Source: three-view drawing plus pictorial views. Frame: mm from the lowest corner of the part. A direction names the side the tool comes from. Give positions to 0.01 mm unless a question says otherwise; leave off trailing zeros. Loops run counter-clockwise (first coordinate to the right, second up) from the corner with the lowest first, then second, coordinate; pieces in that order, holes last. Notation, with made-up numbers: (65.25, -34) - (113.25, -34) arc R19 cw to (113.25, 1) - close; hole circle Ø9 at (47, -31.75). An arc over 180 degrees is marked (long way). One line per item, written item: value.
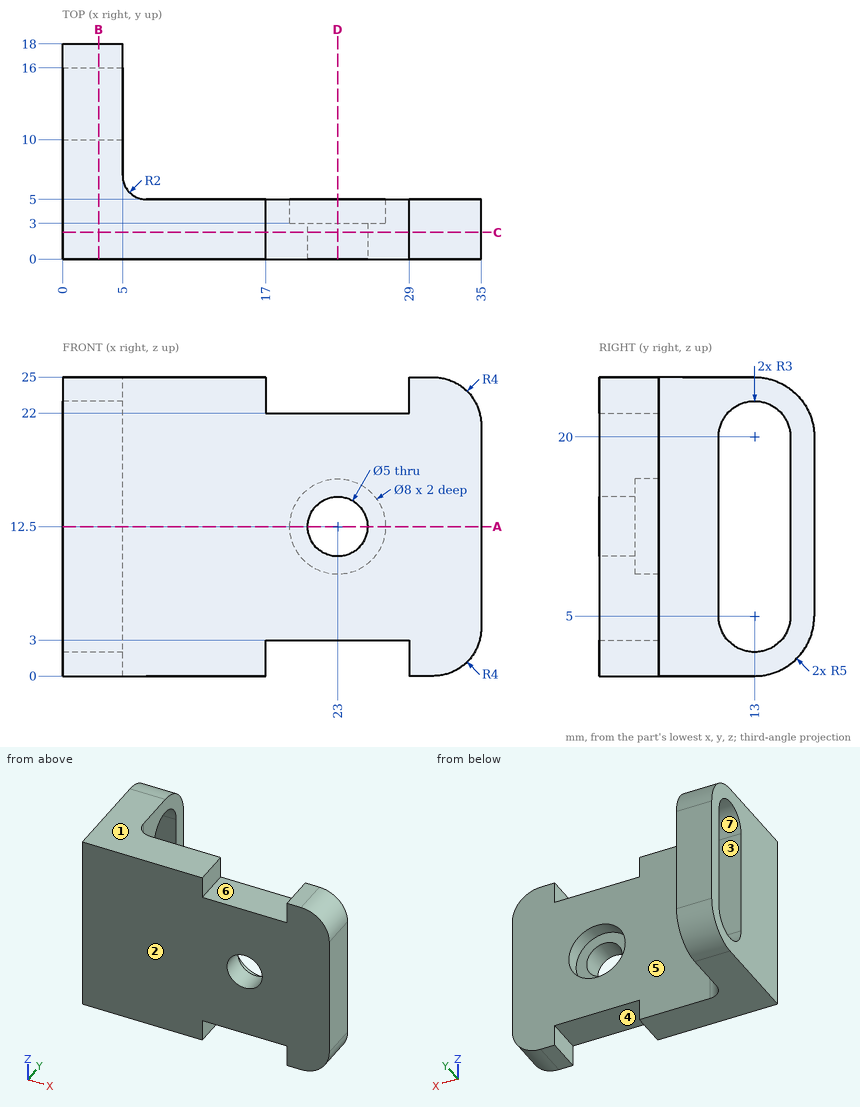
Item 1: Material intervals for L1, parallel to Z at x = 23, y = 1.8; L2, parallel to Z at x = 23, y = 4.4; L3, parallel to Y at x = 8, z = 13, sorted ascending.
Verdict:
L1: z = 3 to 10, 15 to 22
L2: z = 3 to 8.5, 16.5 to 22
L3: y = 0 to 5
Item 2: Draft query along Z for the marked faces 1, 2 and 3. Return one class per face: pulls with the +Z half, pulls with the -Z half, needs draft (parallel to the pull), parting line crosses it, or undercut.
Verdict:
face 1: pulls with the +Z half
face 2: needs draft
face 3: undercut
Item 3: Section B-B, the plane x = 3. Output: boundary loops of the cut face in (y, z), and give its area (3 significant figures).
Verdict:
outline: (0, 0) - (13, 0) arc R5 ccw to (18, 5) - (18, 20) arc R5 ccw to (13, 25) - (0, 25) - close; hole (10, 5) arc R3 ccw to (16, 5) - (16, 20) arc R3 ccw to (10, 20) - close
area: 321 mm^2
Item 4: Section C-C, the plane y = 2.25. Output: boundary loops of the cut face in (x, z).
Verdict:
outline: (0, 0) - (17, 0) - (17, 3) - (29, 3) - (29, 0) - (31, 0) arc R4 ccw to (35, 4) - (35, 21) arc R4 ccw to (31, 25) - (29, 25) - (29, 22) - (17, 22) - (17, 25) - (0, 25) - close; hole circle Ø5 at (23, 12.5)
Item 5: Access query for the marked faces 4, 5, 6 and 7. Directions: +Z, -Z, +X, -X, +Y, -Y. A direction counts if a zero-diameter tool reaches every point of the face in a straight line with its end or side. Return the directions, or none.
Verdict:
face 4: -Z, +Y, -Y
face 5: +Z, -Z, +X, +Y
face 6: +Z, +Y, -Y
face 7: +X, -X
Item 6: Section A-A, the plane z = 12.5. Output: boundary loops of the cut face in (x, y), and give its area (3 significant figures).
Verdict:
outline: (0, 0) - (20.5, 0) - (20.5, 3) - (19, 3) - (19, 5) - (7, 5) arc R2 cw to (5, 7) - (5, 10) - (0, 10) - close; (0, 16) - (5, 16) - (5, 18) - (0, 18) - close; (25.5, 0) - (35, 0) - (35, 5) - (27, 5) - (27, 3) - (25.5, 3) - close
area: 180 mm^2
Item 7: Section D-D, the plane x = 23. Output: boundary loops of the cut face in (y, z).
Verdict:
outline: (0, 3) - (5, 3) - (5, 8.5) - (3, 8.5) - (3, 10) - (0, 10) - close; (0, 15) - (3, 15) - (3, 16.5) - (5, 16.5) - (5, 22) - (0, 22) - close
Item 8: Pin query (flat end, axial travel): P1, Ø2.5, axis at x = 21, y = 3.5, coming from the -Z side; P2, Ø2.5, axis at y = 1.5, z = 23, coming from the +X side; P3, Ø6, axis at x = 29, z = 4.5, coming from the +Y side; P4, Ø1, axis at y = 11, z = 11, coming from the -X side. Return the tip coordinate at first contact, or that it passes through.
Verdict:
P1: stops at z = 3
P2: stops at x = 34.93
P3: stops at y = 5
P4: passes through
